Input: part model. Units: mm. Frame: model coordinates. Give positions to 0.01 mm unless a question says otherwise; leave off trailing zeros. Order: outer loops, then holes, each group sorted by start corner. A loop starts at its lowest first (then second) coordinate and runs counter-clockwise, first axis right, second up. Notation, with made-up numbers: (18.25, 48) -> (52.25, 48) arc R25 ccw to (52.25, 60) -> close; hole circle Ø8 at (-33.5, 89). An arc over 180 degrees is marked (long way). Use a Markdown table: item, result. Add a question column.
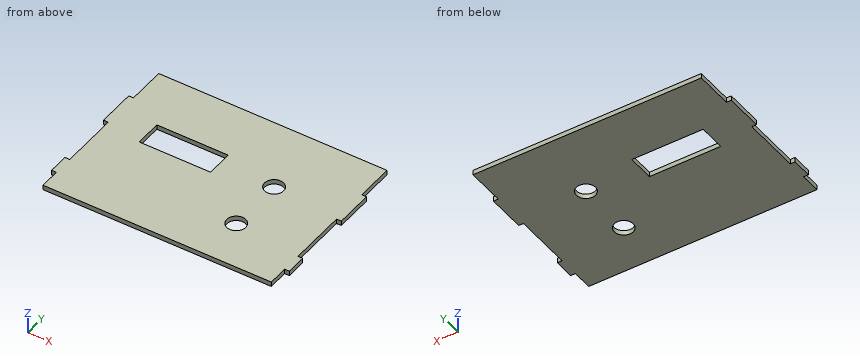
from build123d import *

# Parameters (mm, degrees)
ESQUISSE1_R        = 10
ESQUISSE1_W        = 75
ESQUISSE1_H        = 28
BOSS_EXTRU_1_DEPTH = 5


with BuildPart() as part:
    # Esquisse1 → Boss.-Extru.1 (new body)
    with BuildSketch(Plane.XY):
        Polygon((0, 143.5), (0, 183.5), (240, 183.5), (240, 143.5), (245, 143.5), (245, 103.5), (240, 103.5), (240, 42.333333333), (245, 42.333333333), (245, 21.166666667), (240, 21.166666667), (240, 0), (0, 0), (0, 21.166666667), (-5, 21.166666667), (-5, 42.333333333), (0, 42.333333333), (0, 103.5), (-5, 103.5), (-5, 143.5), align=None)
        with Locations((170, 110)):
            Circle(ESQUISSE1_R, mode=Mode.SUBTRACT)
        with Locations((170, 50)):
            Circle(ESQUISSE1_R, mode=Mode.SUBTRACT)
        with Locations((75, 110)):
            Rectangle(ESQUISSE1_W, ESQUISSE1_H, mode=Mode.SUBTRACT)
    extrude(amount=BOSS_EXTRU_1_DEPTH)


solid = part.part
Q1. Section query B-B (y = 110). Return loops of the section in (x, z).
Q2. Section query A-A (x = 170). Return loops of the section in (y, z), plus the area to 4 significant figures.
Q3. Section query C-C (y = 50). Return loops of the section in (x, z), plus the area to 3 significant figures.
Q4. Section query D-D (z = 4.1). Return loops of the section in (x, y), plus the area to 3 significant figures.
Q5. First-contact query: pin 1 (1.5 mm diameter, centred on y = 11.5, z = 2, fed in from -X); pin 2 (2.5 mm diameter, centred on x = -3, z = 3.5, fed in from +Y); pin 3 (1.5 mm diameter, centred on y = 168.5, z = 2, fed in from +X). Flat tips, straight axial feed; report the tip coordinate or a pass-through.
Q6. Ray query, line 1 (Y direction, x = 170, z = 3.15); line 2 (Y direction, x = 84.5, z = 0.2); line 3 (X direction, y = 157.5, z = 3.4). Return the intervals inside material, ascending.
Solution:
| question | item | result |
|---|---|---|
| 1 | outline | (-5, 0) -> (37.5, 0) -> (37.5, 5) -> (-5, 5) -> close; (112.5, 0) -> (160, 0) -> (160, 5) -> (112.5, 5) -> close; (180, 0) -> (245, 0) -> (245, 5) -> (180, 5) -> close |
| 2 | outline | (0, 0) -> (40, 0) -> (40, 5) -> (0, 5) -> close; (60, 0) -> (100, 0) -> (100, 5) -> (60, 5) -> close; (120, 0) -> (183.5, 0) -> (183.5, 5) -> (120, 5) -> close |
| 2 | area | 717.5 mm² |
| 3 | outline | (0, 0) -> (160, 0) -> (160, 5) -> (0, 5) -> close; (180, 0) -> (240, 0) -> (240, 5) -> (180, 5) -> close |
| 3 | area | 1,100 mm² |
| 4 | outline | (-5, 21.17) -> (0, 21.17) -> (0, 0) -> (240, 0) -> (240, 21.17) -> (245, 21.17) -> (245, 42.33) -> (240, 42.33) -> (240, 103.5) -> (245, 103.5) -> (245, 143.5) -> (240, 143.5) -> (240, 183.5) -> (0, 183.5) -> (0, 143.5) -> (-5, 143.5) -> (-5, 103.5) -> (0, 103.5) -> (0, 42.33) -> (-5, 42.33) -> close; hole (37.5, 96) -> (112.5, 96) -> (112.5, 124) -> (37.5, 124) -> close; hole circle Ø20 at (170, 50); hole circle Ø20 at (170, 110) |
| 4 | area | 41,900 mm² |
| 5 | pin 1 | stops at x = 0 |
| 5 | pin 2 | stops at y = 143.5 |
| 5 | pin 3 | stops at x = 240 |
| 6 | line 1 | y = 0 to 40, 60 to 100, 120 to 183.5 |
| 6 | line 2 | y = 0 to 96, 124 to 183.5 |
| 6 | line 3 | x = 0 to 240 |
